```python
from build123d import *

# Parameters (mm, degrees)
SKETCH_1_W          = 29
SKETCH_1_H          = 35.7
EXTRUDE_1_DEPTH     = 2
SKETCH_2_R          = 1.55
CUT_EXTRUDE_1_DEPTH = 24
SKETCH_4_W          = 24
SKETCH_4_H          = 22.7
CUT_EXTRUDE_2_DEPTH = 10
SKETCH_5_W          = 14
SKETCH_5_H          = 30.7
CUT_EXTRUDE_3_DEPTH = 10
FILLET_START        = -2
FILLET_1_DEPTH      = 4
FILLET_1_2_DEPTH    = 4


with BuildPart() as part:
    # 草图1 → 凸台-拉伸1 (new, symmetric)
    with BuildSketch(Plane.XY):
        Rectangle(SKETCH_1_W, SKETCH_1_H)
    extrude(amount=EXTRUDE_1_DEPTH, both=True)

    # 草图2 → 切除-拉伸1 (cut)
    with BuildSketch(Plane.XY.offset(2)):
        with Locations((10, 14.35)):
            Circle(SKETCH_2_R)
        with Locations((10, -14.35)):
            Circle(SKETCH_2_R)
        with Locations((-10, -14.35)):
            Circle(SKETCH_2_R)
        with Locations((-10, 14.35)):
            Circle(SKETCH_2_R)
    extrude(amount=-CUT_EXTRUDE_1_DEPTH, mode=Mode.SUBTRACT)

    # 草图4 → 切除-拉伸2 (cut)
    with BuildSketch(Plane(origin=(0, 0, -2), x_dir=(-1, 0, 0), z_dir=(0, 0, -1))):
        Rectangle(SKETCH_4_W, SKETCH_4_H)
    extrude(amount=-CUT_EXTRUDE_2_DEPTH, mode=Mode.SUBTRACT)

    # 草图5 → 切除-拉伸3 (cut)
    with BuildSketch(Plane(origin=(0, 0, -2), x_dir=(-1, 0, 0), z_dir=(0, 0, -1))):
        Rectangle(SKETCH_5_W, SKETCH_5_H)
    extrude(amount=-CUT_EXTRUDE_3_DEPTH, mode=Mode.SUBTRACT)

    # 圆角1: read off the stored shape, not the designer's step
    # 圆角1 outline → 圆角1 (cut)
    with BuildSketch(Plane.XY.offset(FILLET_START)):
        with BuildLine():
            Line((14.5, -17.85), (14.5, -15.85))
            ThreePointArc((14.5, -15.85), (13.914213562, -17.264213562), (12.5, -17.85))
            Line((12.5, -17.85), (14.5, -17.85))
        make_face()
        with BuildLine():
            ThreePointArc((12.5, 17.85), (13.914213562, 17.264213562), (14.5, 15.85))
            Line((14.5, 15.85), (14.5, 17.85))
            Line((14.5, 17.85), (12.5, 17.85))
        make_face()
        with BuildLine():
            Line((-14.5, -17.85), (-12.5, -17.85))
            ThreePointArc((-12.5, -17.85), (-13.914213562, -17.264213562), (-14.5, -15.85))
            Line((-14.5, -15.85), (-14.5, -17.85))
        make_face()
        with BuildLine():
            ThreePointArc((-14.5, 15.85), (-13.914213562, 17.264213562), (-12.5, 17.85))
            Line((-12.5, 17.85), (-14.5, 17.85))
            Line((-14.5, 17.85), (-14.5, 15.85))
        make_face()
        with BuildLine():
            ThreePointArc((7, -13.35), (7.585786438, -11.935786438), (9, -11.35))
            Line((9, -11.35), (7, -11.35))
            Line((7, -11.35), (7, -13.35))
        make_face()
        with BuildLine():
            ThreePointArc((-9, -11.35), (-7.585786438, -11.935786438), (-7, -13.35))
            Line((-7, -13.35), (-7, -11.35))
            Line((-7, -11.35), (-9, -11.35))
        make_face()
        with BuildLine():
            Line((7, 11.35), (9, 11.35))
            ThreePointArc((9, 11.35), (7.585786438, 11.935786438), (7, 13.35))
            Line((7, 13.35), (7, 11.35))
        make_face()
        with BuildLine():
            Line((-7, 11.35), (-7, 13.35))
            ThreePointArc((-7, 13.35), (-7.585786438, 11.935786438), (-9, 11.35))
            Line((-9, 11.35), (-7, 11.35))
        make_face()
    extrude(amount=FILLET_1_DEPTH, mode=Mode.SUBTRACT)

    # Fillet 1 2 outline → Fillet 1 2 (add)
    with BuildSketch(Plane.XY.offset(FILLET_START)):
        with BuildLine():
            Line((7, -15.35), (7, -13.35))
            ThreePointArc((7, -13.35), (6.414213562, -14.764213562), (5, -15.35))
            Line((5, -15.35), (7, -15.35))
        make_face()
        with BuildLine():
            ThreePointArc((12, -9.35), (11.414213562, -10.764213562), (10, -11.35))
            Line((10, -11.35), (12, -11.35))
            Line((12, -11.35), (12, -9.35))
        make_face()
        with BuildLine():
            Line((-7, -15.35), (-5, -15.35))
            ThreePointArc((-5, -15.35), (-6.414213562, -14.764213562), (-7, -13.35))
            Line((-7, -13.35), (-7, -15.35))
        make_face()
        with BuildLine():
            ThreePointArc((10, 11.35), (11.414213562, 10.764213562), (12, 9.35))
            Line((12, 9.35), (12, 11.35))
            Line((12, 11.35), (10, 11.35))
        make_face()
        with BuildLine():
            Line((-12, -11.35), (-10, -11.35))
            ThreePointArc((-10, -11.35), (-11.414213562, -10.764213562), (-12, -9.35))
            Line((-12, -9.35), (-12, -11.35))
        make_face()
        with BuildLine():
            ThreePointArc((5, 15.35), (6.414213562, 14.764213562), (7, 13.35))
            Line((7, 13.35), (7, 15.35))
            Line((7, 15.35), (5, 15.35))
        make_face()
        with BuildLine():
            Line((-12, 11.35), (-12, 9.35))
            ThreePointArc((-12, 9.35), (-11.414213562, 10.764213562), (-10, 11.35))
            Line((-10, 11.35), (-12, 11.35))
        make_face()
        with BuildLine():
            ThreePointArc((-7, 13.35), (-6.414213562, 14.764213562), (-5, 15.35))
            Line((-5, 15.35), (-7, 15.35))
            Line((-7, 15.35), (-7, 13.35))
        make_face()
    extrude(amount=FILLET_1_2_DEPTH)


solid = part.part
```
Geometry: final body of the model. Coordinates: model frame, mm. A direction names the side the tool comes from. Round coordinates to 2 decimals unless told otherwise and drop trailing zeros. Loops run counter-clockwise (first coordinate to the right, second up) from the corner with the lowest first, then second, coordinate; pieces in that order, holes last.
Item 1: Mould query, pull axis X, two halves, no side actions, for faces 3 (the cylindrical face through (-13.9, -17.28, -0.03)), 4 (the flat face through (-13, 0, 2)), 5 (the cylindrical face through (11.4, 10.78, -0.03)). Classes: released by +X, released by -X, zero draft, split by the parting line, or undercut.
Checked values:
face 3: released by -X
face 4: zero draft
face 5: undercut
Item 2: Line query: L1, parallel to Y at x = 10, z = -0.85; L2, parallel to Y at x = -4.75, z = -0.3. Output: solid intervals per line, ascending.
Checked values:
L1: y = -17.85 to -15.9, -12.8 to -11.35, 11.35 to 12.8, 15.9 to 17.85
L2: y = -17.85 to -15.35, 15.35 to 17.85
Item 3: Section D-D, the plane y = 14.35. Output: boundary loops of the cut face in (x, z).
Checked values:
outline: (-14.5, -2) - (-11.55, -2) - (-11.55, 2) - (-14.5, 2) - close; (-8.45, -2) - (-6.73, -2) - (-6.73, 2) - (-8.45, 2) - close; (6.73, -2) - (8.45, -2) - (8.45, 2) - (6.73, 2) - close; (11.55, -2) - (14.5, -2) - (14.5, 2) - (11.55, 2) - close
Item 4: Contact query for flat-ended pins moving along their axis: P1, Ø2.5, axis at x = 10, y = 14.35, coming from the -Z side; P2, Ø2, axis at x = 7, y = 12.5, coming from the +Z side. Output: stop coordinate, or through.
Checked values:
P1: passes through
P2: stops at z = 2
Item 5: Section C-C, the plane y = 6.5. Output: boundary loops of the cut face in (x, z).
Checked values:
outline: (-14.5, -2) - (-12, -2) - (-12, 2) - (-14.5, 2) - close; (12, -2) - (14.5, -2) - (14.5, 2) - (12, 2) - close
Item 6: Reachability of faces 1 (the flat face through (14.5, 0, 0)), 2 (the cylindrical face through (11.43, -10.75, -0.03)) from +Z, -Z, +X, -X, +Y, -Y: full face, straight path, thin tool, end or side. Return the list, or none.
Checked values:
face 1: +Z, -Z, +X, +Y, -Y
face 2: +Z, -Z
Item 7: Section B-B, the plane x = -2. Output: boundary loops of the cut face in (y, z).
Checked values:
outline: (-17.85, -2) - (-15.35, -2) - (-15.35, 2) - (-17.85, 2) - close; (15.35, -2) - (17.85, -2) - (17.85, 2) - (15.35, 2) - close
Item 8: Section A-A, the plane z = 1.5. State how many separate pieces and enclosed holes the cut face has, plus the area to 3 significant figures.
Checked values:
separate pieces: 1
enclosed holes: 5
area: 348 mm2
